Here's how the part is built. I have some questions about the finished solid (model axes, mm). A direction names the side the tool comes from. Coordinates: 2 decimals unless noted, no trailing zeros. Loops run counter-clockwise (first coordinate to the right, second up) from the corner with the lowest first, then second, coordinate; pieces in that order, holes last. Notation, with made-up numbers: (82, 51.25) -> (105, 51.25) arc R27 ccw to (105, 74.25) -> close; hole circle Ø3 at (19, 59.25). An arc over 180 degrees is marked (long way). Answer as a JSON object with one key per item and string values. Group by question number.
1) Which directions (+Z, -Z, +X, -X, +Y, -Y) give clear straight access to the entire face, cutting with the end or side of a thin tool? Please do faces 4 (the cylindrical face through (10.526, 0.054, 0.986)), 5 (the flat face through (-12, -7, 1)), 6 (the flat face through (7.75, -9, 1)).
2) I need wall thicknesses on probe 1 along Y at (x, z) = (11.75, 0.9) (3 decimals); probe 2 along X at (y, z) = (-0.5, 1.55); probe 3 along Y at (x, z) = (10, 0.1). Which ranges of each line are inside material? Lowest first, please. Write a range as [from, to].
3) I'm going to push flat-ended pins straight in: pin 1 (1 mm diameter, centred on x = 10.5, z = 0.5, fed in from -Y); pin 2 (0.6 mm diameter, centred on y = -9, z = 1, fed in from +X); pin 3 (1.5 mm diameter, centred on x = -11.75, y = 0, fed in from +Z). Where does each tip first touch, or does it pass through?
4) If we mould it in two halves opening along X, with no side actions, what happens to faces 1 (the cylindrical face through (-12.974, 0.054, 0.986)), 2 (the flat face through (-15.75, -4, 1)), 3 (the flat face through (12, -7, 1))? For each: +X half, -X half, draft (parallel to the pull), parting line (faces both ways), or undercut.
5) I want a section at D-D (y = -8). Write out the boundary of the cut face in (x, z).
6) I want a section at A-A (z = 0.45). Write out the boundary of the cut face in (x, y) (3 decimals), then the cut area to 3 significant figures.
7) I want a section at B-B (y = 0). Write out the boundary of the cut face in (x, z) (3 decimals).
8) I want a section at C-C (x = 10). Write out the boundary of the cut face in (y, z), then the cut area to 3 significant figures.
```python
from build123d import *

# Parameters (mm, degrees)
SKETCH1_R       = 1.225
MAIN_BODY_DEPTH = 2


with BuildPart() as part:
    # Sketch1 → Main Body (new body)
    with BuildSketch(Plane.XY):
        with BuildLine():
            Line((-15.75, -7), (-7.75, -7))
            Line((-7.75, -7), (-7.75, -11))
            Line((-7.75, -11), (7.75, -11))
            Line((7.75, -11), (7.75, -7))
            Line((7.75, -7), (15.75, -7))
            Line((15.75, -7), (15.75, -1))
            ThreePointArc((15.75, -1), (14.578427125, 1.828427125), (11.75, 3))
            Line((11.75, 3), (-11.75, 3))
            ThreePointArc((-11.75, 3), (-14.578427125, 1.828427125), (-15.75, -1))
            Line((-15.75, -1), (-15.75, -7))
        make_face()
        with Locations((-11.75, 0)):
            Circle(SKETCH1_R, mode=Mode.SUBTRACT)
        with Locations((11.75, 0)):
            Circle(SKETCH1_R, mode=Mode.SUBTRACT)
    extrude(amount=MAIN_BODY_DEPTH)


solid = part.part
```
Determined:
{
 "1": {"face 4": "+Z, -Z", "face 5": "+Z, -Z, -X, -Y", "face 6": "+Z, -Z, +X, -Y"},
 "2": {"probe 1": "[-7, -1.225], [1.225, 3]", "probe 2": "[-15.72, -12.87], [-10.63, 10.63], [12.87, 15.72]", "probe 3": "[-7, 3]"},
 "3": {"pin 1": "y = -7", "pin 2": "x = 7.75", "pin 3": "through"},
 "4": {"face 1": "undercut", "face 2": "-X half", "face 3": "draft"},
 "5": {"outline": "(-7.75, 0) -> (7.75, 0) -> (7.75, 2) -> (-7.75, 2) -> close"},
 "6": {"outline": "(-15.75, -7) -> (-7.75, -7) -> (-7.75, -11) -> (7.75, -11) -> (7.75, -7) -> (15.75, -7) -> (15.75, -1) arc R4 ccw to (11.75, 3) -> (-11.75, 3) arc R4 ccw to (-15.75, -1) -> close; hole circle Ø2.45 at (-11.75, 0); hole circle Ø2.45 at (11.75, 0)", "area": "361 mm^2"},
 "7": {"outline": "(-15.623, 0) -> (-12.975, 0) -> (-12.975, 2) -> (-15.623, 2) -> close; (-10.525, 0) -> (10.525, 0) -> (10.525, 2) -> (-10.525, 2) -> close; (12.975, 0) -> (15.623, 0) -> (15.623, 2) -> (12.975, 2) -> close"},
 "8": {"outline": "(-7, 0) -> (3, 0) -> (3, 2) -> (-7, 2) -> close", "area": "20.0 mm^2"}
}
